Autodesk Inventor part; units mm, degrees
ref_plane "YZ Plane" through (0, 0, 0) normal (1, 0, 0) x (0, 1, 0)
ref_plane "XZ Plane" through (0, 0, 0) normal (0, 1, 0) x (-1, 0, 0)
ref_plane "XY Plane" through (0, 0, 0) normal (0, 0, 1) x (1, 0, 0)
sketch "Szkic1" plane through (0, 0, 0) normal (0, 1, 0) x (-1, 0, 0)
  line L0 (0, 0) -> (-50, 0)
  line L1 (-50, 0) -> (-50, -50)
  line L2 (-50, -50) -> (0, -50)
  line L3 (0, -50) -> (0, 0)
  line L4 (0, -50) -> (-8, -50)
  line L5 (-8, -50) -> (-8, -30)
  line L6 (-8, -30) -> (0, -30)
  line L7 (0, -30) -> (0, -50)
  line L8 (-50, -50) -> (-42, -50)
  line L9 (-42, -50) -> (-42, -30)
  line L10 (-42, -30) -> (-50, -30)
  line L11 (-50, -30) -> (-50, -50)
  dimension "d0" = 50
  dimension "d1" = 50
  dimension "d2" = 8
  dimension "d3" = 20
  dimension "d4" = 8
  dimension "d5" = 20
extrude "Wyciągnięcie proste1" add sketch "Szkic1" along normal blind 2 contours L3 L6 L5 L2 L9 L10 L1 L0
sketch "Szkic4" plane through (0, 2, 0) normal (0, 1, 0) x (1, 0, 0)
  line L0 (42, 50) -> (8, 50)
  line L1 (12.0571, 48.5) -> (42.467, 48.5)
  line L2 (42, 30) -> (42, 50)
  line L3 (42, 50) -> (8, 50)
  line L4 (8, 50) -> (8, 48.5)
  line L5 (8, 48.5) -> (42, 48.5)
  line L6 (42, 48.5) -> (42, 50)
  circle A0 centre (39.467, 46.75) radius 0.85
  circle A1 centre (15.0571, 46.75) radius 0.85
  arc A2 (48.301, 27.6749) -> (46.5, 27.9321) centre (47.25, 26.75) ccw
  point P0 (0, 0)
  point P1 (42, 48.5)
extrude "Wyciągnięcie proste3" cut sketch "Szkic4" against normal through all
sketch "Szkic6" plane through (0, 0, -30) normal (-1, 0, 0) x (0, 0, 1)
  line L0 (0, 0) -> (30, 0)
  line L1 (30, 0) -> (30, 2)
  line L2 (0, 2) -> (30, 2)
  line L3 (0, 0) -> (0, 2)
  line L4 (20.8419, 34.4275) -> (27.9622, -2)
  line L5 (27.9622, -2) -> (30, -2)
  line L6 (30, -2) -> (22.8048, 34.8111)
  line L7 (22.8048, 34.8111) -> (20.8419, 34.4275)
  point P0 (27.1803, 2)
  point P1 (27.5712, 0)
extrude "Wyciągnięcie proste5" cut sketch "Szkic6" against normal through all contours L4 L2 L6 L0 | L6 L2 L1 L0
sketch "Szkic7" plane through (0, 0, 0) normal (0, -1, 0) x (1, 0, 0)
  line L0 (50, -2.4288) -> (0, -2.4288)
  line L1 (0, -30) -> (0, -2.4288)
  line L2 (8, -30) -> (0, -30)
  line L3 (8, -48.5) -> (8, -30)
  line L4 (8, -48.5) -> (42, -48.5)
  line L5 (42, -30) -> (42, -48.5)
  line L6 (50, -30) -> (42, -30)
  line L7 (50, -2.4288) -> (50, -30)
  circle A0 centre (39.467, -46.75) radius 0.85
  circle A1 centre (15.0571, -46.75) radius 0.85
  line L8 (4, -10.1324) -> (0, -10.1324)
  line L9 (50, -10.1324) -> (45.5, -10.1324)
  line L10 (50, -10.1324) -> (42, -10.1324)
  line L11 (42, -10.1324) -> (42, -2.4288)
  line L12 (42, -2.4288) -> (50, -2.4288)
  line L13 (50, -2.4288) -> (50, -10.1324)
  line L14 (0, -2.4288) -> (8, -2.4288)
  line L15 (8, -2.4288) -> (8, -10.1324)
  line L16 (8, -10.1324) -> (0, -10.1324)
  line L17 (0, -10.1324) -> (0, -2.4288)
  point P0 (0, 0)
  dimension "d16" = 8
  dimension "d17" = 8
extrude "Wyciągnięcie proste6" cut sketch "Szkic7" against normal through all contours L7 L9 L10 L11 L0 | L15 L16 L8 L1 L0
fillet "Zaokrąglenie1" radius 1 4 edges at (0, 1, -30) (0, 1, -10.1324) (50, 1, -10.1324) (50, 1, -30)
sketch "Szkic9" plane through (0, 2, 0) normal (0, 1, 0) x (1, 0, 0)
  circle A0 centre (15.0571, 46.75) radius 0.85
  circle A1 centre (39.467, 46.75) radius 0.85
  point P0 (0, 0)
extrude "Wyciągnięcie proste8" add sketch "Szkic9" against normal up to surface (2 mm away)
sketch "Szkic10" plane through (0, 0, 0) normal (0, -1, 0) x (1, 0, 0)
  circle A0 centre (17.4483, -46.15) radius 0.6
  circle A1 centre (39.0758, -46.15) radius 0.6
  circle A2 centre (13.5571, -35.5) radius 0.6
  circle A3 centre (46.2335, -26.3) radius 1.35
  circle A4 centre (47.3, -13.0919) radius 1.35
  circle A5 centre (3, -27) radius 1.4
  circle A6 centre (3, -27) radius 1.55
  circle A7 centre (46.2335, -26.3) radius 1.55
  circle A8 centre (47.3, -13.0919) radius 1.55
  circle A9 centre (13.5571, -35.5) radius 0.85
  circle A10 centre (17.4483, -46.15) radius 0.85
  circle A11 centre (39.0758, -46.15) radius 0.85
  point P0 (0, 0)
  dimension "d25" = 3.1
  dimension "d26" = 1.7
extrude "Wyciągnięcie proste9" cut sketch "Szkic10" against normal through all contours A0 | A1 | A2 | A3 | A7 | A9 | A10 | A11
sketch "Szkic11" plane through (0, 0, 0) normal (0, -1, 0) x (1, 0, 0)
  circle A0 centre (47.3, -13.0919) radius 1.55
  circle A1 centre (46.2335, -26.3) radius 1.55
  circle A2 centre (3, -27) radius 1.55
  circle A3 centre (13.5571, -35.5) radius 0.85
  circle A4 centre (17.4483, -46.15) radius 0.85
  circle A5 centre (39.0758, -46.15) radius 0.85
  point P0 (0, 0)
hole "Otwór1" at (46.2335, 0, -26.3) direction (0, 1, 0) diameter 5 depth 1.1
hole "Otwór2" at (13.5571, 0, -35.5) at (17.4483, 0, -46.15) at (39.0758, 0, -46.15) direction (0, 1, 0) diameter 3 depth 1
sketch "Szkic12" plane through (0, 0, 0) normal (0, -1, 0) x (1, 0, 0)
  line L0 (49, -10.1324) -> (42, -10.1324)
  line L1 (8, -10.1324) -> (1, -10.1324)
  line L2 (50, -11.1324) -> (50, -29)
  line L3 (0, -29) -> (0, -11.1324)
  line L4 (50, -2.4288) -> (37, -2.4288)
  line L5 (37, -2.4288) -> (37, -10.1324)
  line L6 (37, -10.1324) -> (50, -10.1324)
  line L7 (50, -10.1324) -> (50, -2.4288)
  line L8 (0, -2.4288) -> (13, -2.4288)
  line L9 (13, -2.4288) -> (13, -10.1324)
  line L10 (13, -10.1324) -> (0, -10.1324)
  line L11 (0, -10.1324) -> (0, -2.4288)
  line L12 (42, -2.4288) -> (8, -2.4288)
  point P0 (0, 0)
  dimension "d43" = 13
  dimension "d44" = 13
extrude "Wyciągnięcie proste10" cut sketch "Szkic12" against normal through all
fillet "Zaokrąglenie2" radius 1 2 edges at (13, 1, -10.1324) (37, 1, -10.1324)
sketch "Szkic13" plane through (0, 2, 0) normal (0, 1, 0) x (1, 0, 0)
  line L0 (10.7953, -1.4378) -> (38.6557, -1.4378)
  line L1 (38.6557, -1.4378) -> (38.6557, 3.4288)
  line L2 (38.6557, 3.4288) -> (10.7953, 3.4288)
  line L3 (10.7953, 3.4288) -> (10.7953, -1.4378)
  line L4 (37, 2.4288) -> (13, 2.4288)
  point P0 (0, 0)
  dimension "d48" = 1
extrude "Wyciągnięcie proste11" cut sketch "Szkic13" against normal through all
fillet "Zaokrąglenie3" radius 1 2 edges at (13, 1, -3.4288) (37, 1, -3.4288)
fillet "Zaokrąglenie4" radius 4 1 edges at (25, 0, -48.5)
chamfer "Faza1" distance 0.5 angle 45 4 edges at (16.5983, 1, -46.15) (38.2258, 1, -46.15) (44.6835, 1.1, -26.3) (12.7071, 1, -35.5)
sketch "Szkic14" plane through (0, 0, 0) normal (0, -1, 0) x (1, 0, 0)
  circle A0 centre (2.8, -24.8689) radius 1.4
  point P0 (0, 0)
hole "Otwór3" at (2.8, 0, -24.8689) direction (0, 1, 0) diameter 3 depth 2 counterbore diameter 5 counterbore depth 1
chamfer "Faza2" distance 0.5 angle 45 1 edges at (2.8, 1, -23.3689)
properties part number "podstawa_v2"
For this review, take the finished solid that the model builds, in its own axes (mm). A direction names the side the tool comes from. Coordinates: 2 decimals unless noted, no trailing zeros. Order: outer loops, then holes, each group sorted by start corner. A loop starts at its lowest first (then second) coordinate and runs counter-clockwise, first axis right, second up. Notation, with made-up numbers: (-0.5, 17) -> (47.5, 17) arc R14 ccw to (47.5, 35) -> close; hole circle Ø11 at (41, -17.5). An arc over 180 degrees is marked (long way). Answer as CSV lines item,"result".
Q1. For faces 4 (the face through (7, 1, -10.132)), 5 (the face through (4, 1, -23)), 6 (the face through (45, 1, -30)), list the 3-axis set-ups (+Z, -Z, +X, -X, +Y, -Y) from which the entire face can be reached by the end or side of a thin tool; tool diameter is ignored.
Model answer:
face 4,"+Z, -X, +Y, -Y"
face 5,"-Y"
face 6,"-Z, +X, +Y, -Y"
Q2. Clearance check with flat-ended pins moving along their axes: pin 1 Ø5 at (x, z) = (22, -10) entering from -Y; pin 2 Ø2 at (x, z) = (13.56, -35.5) entering from -Y; pin 3 Ø0.6 at (y, z) = (1, -42) entering from +X; pin 4 Ø2.5 at (x, z) = (17.45, -46.15) entering from -Y. State where each tip first meets the part, or that it passes through.
Model answer:
pin 1,"stops at y = 0"
pin 2,"stops at y = 1.35"
pin 3,"stops at x = 42"
pin 4,"stops at y = 1.1"
Q3. We need section A-A (z = -35.5). State the section outline as (x, y) points, plus the area to 4 significant figures.
Model answer:
outline,"(8, 0) -> (12.06, 0) -> (12.06, 1) -> (12.21, 1) -> (12.71, 1.5) -> (12.71, 2) -> (8, 2) -> close; (14.41, 1.5) -> (14.91, 1) -> (15.06, 1) -> (15.06, 0) -> (42, 0) -> (42, 2) -> (14.41, 2) -> close"
area,"63.05 mm2"
Q4. Draft analysis for pull direction X (two halves, no side actions). For faces 1 (the face through (42, 1, -39)), 2 (the face through (2.69, 0.51, -22.37)), 3 (the face through (25, 0, -24)), state which applies: released by +X, released by -X, zero draft, split by the parting line, or undercut.
Model answer:
face 1,"released by +X"
face 2,"undercut"
face 3,"zero draft"
Q5. We need section B-B (x = 2.8). State the section outline as (y, z) points, plus the area to 3 significant figures.
Model answer:
outline,"(0, -30) -> (2, -30) -> (2, -26.37) -> (1.5, -26.37) -> (1, -26.87) -> (1, -27.37) -> (0, -27.37) -> close; (0, -22.37) -> (1, -22.37) -> (1, -22.87) -> (1.5, -23.37) -> (2, -23.37) -> (2, -10.13) -> (0, -10.13) -> close"
area,"31.5 mm2"
Q6. We need section C-C (y = 0.35). State the section outline as (x, z) points.
Model answer:
outline,"(0, -29) arc R1 ccw to (1, -30) -> (8, -30) -> (8, -46.67) -> (16.04, -46.67) arc R1.5 cw (long way) to (18.85, -46.67) -> (37.67, -46.67) arc R1.5 cw (long way) to (40.48, -46.67) -> (42, -46.67) -> (42, -30) -> (49, -30) arc R1 ccw to (50, -29) -> (50, -11.13) arc R1 ccw to (49, -10.13) -> (38, -10.13) arc R1 cw to (37, -9.13) -> (37, -4.43) arc R1 ccw to (36, -3.43) -> (14, -3.43) arc R1 ccw to (13, -4.43) -> (13, -9.13) arc R1 cw to (12, -10.13) -> (1, -10.13) arc R1 ccw to (0, -11.13) -> close; hole circle Ø5 at (2.8, -24.87); hole circle Ø3 at (13.56, -35.5); hole circle Ø5 at (46.23, -26.3)"
Q7. Wall thickness on line 1 along X through (y, z) = (0.55, -45.5); line 2 along X through (y, z) = (0.35, -26.3); line 3 along X through (y, z) = (0.3, -35.5): over which ranges is each line inside the solid? List them lowest first. Write a range as [from, to].
Model answer:
line 1,"x = [8, 16.1], [18.8, 37.72], [40.43, 42]"
line 2,"x = [0, 0.75], [4.85, 43.73], [48.73, 50]"
line 3,"x = [8, 12.06], [15.06, 42]"
Q8. We need section D-D (z = -46.15). State the section outline as (x, y) points.
Model answer:
outline,"(8, 0.16) -> (15.95, 0.16) -> (15.95, 1) -> (16.1, 1) -> (16.6, 1.5) -> (16.6, 2) -> (8, 2) -> close; (18.3, 1.5) -> (18.8, 1) -> (18.95, 1) -> (18.95, 0.16) -> (37.58, 0.16) -> (37.58, 1) -> (37.73, 1) -> (38.23, 1.5) -> (38.23, 2) -> (18.3, 2) -> close; (39.93, 1.5) -> (40.43, 1) -> (40.58, 1) -> (40.58, 0.16) -> (42, 0.16) -> (42, 2) -> (39.93, 2) -> close"
